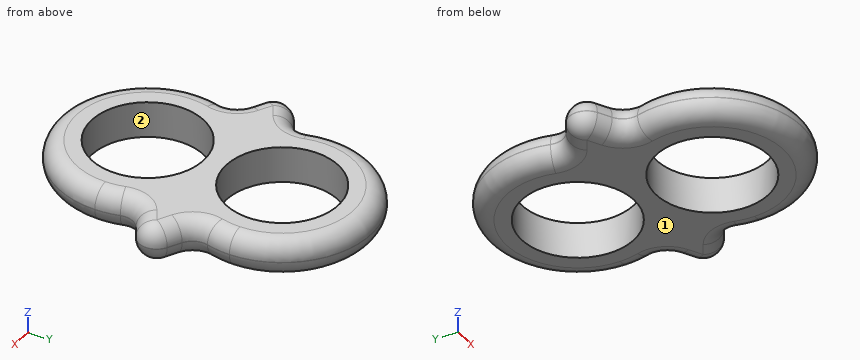
```python
from build123d import *

# Parameters (mm, degrees)
F1_DEPTH = 7.075
F3_DEPTH = 7.075
F4_D     = 22.075
F4_DEPTH = 35.375
F4_TIP   = 6.6319990825
F5_F1_R  = 3.5
F5_F2_R  = 3.5
F5_F3_R  = 3.5


# Not quite as in the source:
# - a pattern or mirror of a feature is missing from the dataset's text; its kind, count and spacing are read off the source's solid


with BuildPart() as f1:
    # F0 (on Top) → F1 (new body)
    with BuildSketch(Plane.XY):
        with BuildLine():
            ThreePointArc((11.7153745139, 0), (15.9885748895, 5.8855447852), (17.5, 13))
            ThreePointArc((17.5, 13), (-7.1144552148, 28.9885748895), (-11.7153745139, 0))
            ThreePointArc((-11.7153745139, 0), (0, 4.5), (11.7153745139, 0))
        make_face()
        with BuildLine():
            ThreePointArc((11.7153745139, 0), (0, -4.5), (-11.7153745139, 0))
            ThreePointArc((-11.7153745139, 0), (-7.1144552148, -28.9885748895), (17.5, -13))
            ThreePointArc((17.5, -13), (15.9885748895, -5.8855447852), (11.7153745139, 0))
        make_face()
        with BuildLine():
            ThreePointArc((11.7153745139, 0), (0, 4.5), (-11.7153745139, 0))
            ThreePointArc((-11.7153745139, 0), (0, -4.5), (11.7153745139, 0))
        make_face()
    extrude(amount=F1_DEPTH)

    # F2 (on Top) → F3 (join)
    with BuildSketch(Plane.XY):
        Polygon((26.25, 0), (0, 15.1554445662), (0, -15.1554445662), align=None)
    f3 = extrude(amount=F3_DEPTH)

    # F3_copies: F3 across plane
    add(f3.mirror(Plane(origin=(0, 0, 0), x_dir=(0, 0, -1), z_dir=(-1, 0, 0))))

    # F4
    with Locations(Plane(origin=(0, 0, 0), x_dir=(1, 0, 0), z_dir=(0, 0, -1))):
        with Locations((0, -13), (0, 13)):
            Hole(F4_D / 2, depth=F4_DEPTH)
            with Locations((0, 0, -(F4_DEPTH + F4_TIP / 2))):  # 118° drill point
                Cone(0, F4_D / 2, F4_TIP, mode=Mode.SUBTRACT)

    # F5: fillet of radius 3.5 on 14 edges, made by hand

    # F5_f1
    f5_f1_edges = [f1.edges().sort_by_distance(p)[0] for p in [
        (16.0023148685, -5.9165037693, 3.5375),
        (-16.0023148685, 5.9165037693, 3.5375),
        (16.0023148685, 5.9165037693, 3.5375),
        (-16.0023148685, -5.9165037693, 3.5375),
    ]]
    fillet(f5_f1_edges, radius=F5_F1_R)

    # F5_f2
    f5_f2_edges = [f1.edges().sort_by_distance(p)[0] for p in [
        (26.25, 0, 3.5375),
        (-26.25, 0, 3.5375),
    ]]
    fillet(f5_f2_edges, radius=F5_F2_R)

    # F5_f3
    f5_f3_edges = [f1.edges().sort_by_distance(p)[0] for p in [
        (19.7579861931, -3.748165919, 0),
        (19.7579861931, -3.748165919, 7.075),
        (0, 30.5, 0),
        (0, 30.5, 7.075),
        (0, -30.5, 0),
        (0, -30.5, 7.075),
        (19.7579861931, 3.748165919, 0),
        (19.7579861931, 3.748165919, 7.075),
        (22.75, 0, 7.075),
        (17.03013711, 6.1624015307, 7.075),
        (22.75, 0, 0),
        (17.03013711, 6.1624015307, 0),
        (-17.03013711, -6.1624015307, 7.075),
        (17.03013711, -6.1624015307, 7.075),
        (-17.03013711, -6.1624015307, 0),
        (17.03013711, -6.1624015307, 0),
        (-17.03013711, 6.1624015307, 7.075),
        (-17.03013711, 6.1624015307, 0),
    ]]
    fillet(f5_f3_edges, radius=F5_F3_R)


solid = f1.part
```
Check sheet for the modelled part. Datum: model origin and axes. Units: mm. Face numbers are marked on the shaded views. Round coordinates to 2 decimals unless told otherwise and drop trailing zeros. Answer in a Markdown table with one row per item.
(1) Section check A-A on x = 0. Give the number of separate pieces and of enclosed holes in the cut face, plus the area to 3 significant figures.
Findings:
| item | result |
|---|---|
| separate pieces | 3 |
| enclosed holes | 0 |
| area | 109 mm^2 |
(2) Gauge pin test, flat ends, axial feed: pin 1 (1 mm diameter, centred on y = -10, z = 1.5, fed in from -X); pin 2 (3 mm diameter, centred on x = 15, z = 1, fed in from -Y); pin 3 (2 mm diameter, centred on x = -15.5, z = 2.5, fed in from -Y). Record the tip position at first contact, or that the pin passes through.
Findings:
| item | result |
|---|---|
| pin 1 | stops at x = -16.91 |
| pin 2 | stops at y = -23.12 |
| pin 3 | stops at y = -22.6 |
(3) Material ranges on line 1 along Y through (x, z) = (0, 3.75); line 2 along Y through (x, z) = (0, 1.75); line 3 along X through (y, z) = (-13.5, 3.5), recorded low to high. Write a range as from..to.
Findings:
| item | result |
|---|---|
| line 1 | y = -30.5..-24.04, -1.96..1.96, 24.04..30.5 |
| line 2 | y = -30.03..-24.04, -1.96..1.96, 24.04..30.03 |
| line 3 | x = -17.49..-11.03, 11.03..17.49 |
(4) Draft check along Y on the marked faces 1 and 2. Enter one of: +Y half, -Y half, draft (parallel to the pull), parting line (faces both ways), or undercut.
Findings:
| item | result |
|---|---|
| face 1 | draft |
| face 2 | undercut |
